```python
from build123d import *

# Parameters (mm, degrees)
SKE_W          = 3
SKE_H          = 24
CHAMFER1_SIZE  = 0.321539
CHAMFER1_SIZE2 = 1.2


with BuildPart() as part:
    # Ske → Base-Rev (revolve)
    with BuildSketch(Plane.XY, mode=Mode.PRIVATE) as base_rev_sk:
        with Locations((1.5, 12)):
            Rectangle(SKE_W, SKE_H)
    revolve(base_rev_sk.sketch.rotate(Axis((0, 0, 0), (0, 1, 0)), 90), axis=Axis((0, 0, 0), (0, 1, 0)))

    # Chamfer2: read off the stored shape, not the designer's step
    # Chamfer2 outline → Chamfer2 (revolve, cut)
    with BuildSketch(Plane.XY):
        Polygon((3, 1.2), (2.678460969, 0), (3, 0), align=None)
    revolve(axis=Axis((0, 0, 0), (0, 1, 0)), mode=Mode.SUBTRACT)

    # Chamfer1: size read off the stored shape
    # Chamfer1
    chamfer1_edges = [part.edges().sort_by_distance(p)[0] for p in [
        (0, 24, 3),
    ]]
    chamfer1_side = [part.faces().sort_by_distance(p)[0] for p in [
        (0, 24, 0),
    ]]
    chamfer(chamfer1_edges, length=CHAMFER1_SIZE, length2=CHAMFER1_SIZE2, reference=chamfer1_side[0])


solid = part.part
```
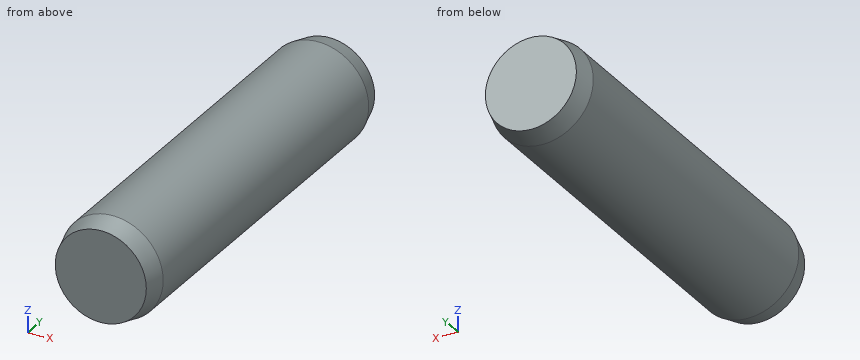
Model file for the job. Use its own axes, mm. Coordinates: 2 decimals unless noted, no trailing zeros. Write each loop counter-clockwise with the first axis right and the second up, starting at its lowest first coordinate (ties: lowest second). Pieces come first, ordered by that corner, then holes. Notation, with made-up numbers: (8, 20.5) - (50, 20.5) arc R26 cw to (50, 41.5) - close; hole circle Ø9 at (-1.5, 81.25). An arc over 180 degrees is marked (long way). Use a Markdown table: item, result. Add a question column.
Item 1: Band-saw the part on A-A, the plane y = 9.75. Write the cut outline in (x, z), and give its area (3 significant figures).
Item 2: Drill centre lines: line 1 along X through (y, z) = (20, -0.1); line 2 along X through (y, z) = (10, -1.35); line 3 along Z through (x, y) = (2.1, 19). Where is each one in solid material? Low to high.
Item 3: Drop flat-ended pins along their axis: pin 1 (1 mm diameter, centred on y = 21, z = 1, fed in from +X); pin 2 (3 mm diameter, centred on y = 6, z = 1.5, fed in from -X). Give the stop position or say it passes through.
A:
| question | item | result |
|---|---|---|
| 1 | outline | circle Ø6 at (0, 0) |
| 1 | area | 28.3 mm² |
| 2 | line 1 | x = -3 to 3 |
| 2 | line 2 | x = -2.68 to 2.68 |
| 2 | line 3 | z = -2.14 to 2.14 |
| 3 | pin 1 | stops at x = 2.96 |
| 3 | pin 2 | stops at x = -3 |
